Part model, mm, in its own coordinate system. A direction names the side the tool comes from. Round coordinates to 2 decimals unless told otherwise and drop trailing zeros. Order: outer loops, then holes, each group sorted by start corner. A loop starts at its lowest first (then second) coordinate and runs counter-clockwise, first axis right, second up. Notation, with made-up numbers: M -4.5,-32.5 L 23.5,-32.5 A27 cw 23.5,-14.5 Z; hole C 48,22.5 d2. An arc over 180 degrees is marked long. One line per question, with ' | ' between items.
from build123d import *

# Parameters (mm, degrees)
SKETCH1_R           = 17.000673514
SKETCH1_R_2         = 12
BOSS_EXTRUDE1_DEPTH = 15
BOSS_EXTRUDE2_DEPTH = 15
BOSS_EXTRUDE3_DEPTH = 15


with BuildPart() as part:
    # Sketch1 → Boss-Extrude1 (new body)
    with BuildSketch(Plane(origin=(0, 0, 0), x_dir=(1, 0, 0), z_dir=(0, 1, 0))):
        Circle(SKETCH1_R)
        Circle(SKETCH1_R_2, mode=Mode.SUBTRACT)
    extrude(amount=BOSS_EXTRUDE1_DEPTH)

    # Sketch2 → Boss-Extrude2 (add)
    with BuildSketch(Plane(origin=(0, 15, 0), x_dir=(1, 0, 0), z_dir=(0, 1, 0))):
        with BuildLine():
            Line((0, 17.000673514), (25, 17.000673514))
            Line((25, 17.000673514), (25, -17.000673514))
            Line((25, -17.000673514), (0, -17.000673514))
            ThreePointArc((0, -17.000673514), (17.000673514, 0), (0, 17.000673514))
        make_face()
    extrude(amount=-BOSS_EXTRUDE2_DEPTH)

    # Sketch3 → Boss-Extrude3 (add)
    with BuildSketch(Plane(origin=(0, 0, 0), x_dir=(-1, 0, 0), z_dir=(0, -1, 0))):
        with BuildLine():
            ThreePointArc((-29.598035728, 0), (-39.849298386, -24.748737342), (-64.598035728, -35))
            Line((-64.598035728, -35), (-64.598035728, -43.228194221))
            ThreePointArc((-64.598035728, -43.228194221), (-34.031086456, -30.566949272), (-21.369841507, 0))
            ThreePointArc((-21.369841507, 0), (-34.031086456, 30.566949272), (-64.598035728, 43.228194221))
            Line((-64.598035728, 43.228194221), (-64.598035728, 35))
            ThreePointArc((-64.598035728, 35), (-39.849298386, 24.748737342), (-29.598035728, 0))
        make_face()
    extrude(amount=-BOSS_EXTRUDE3_DEPTH)


solid = part.part
1) Saw through at D-D (z = -34). List the corners of the cut face in (x, y), plus the area to 3 significant figures.
The answers:
outline: M 37.9,0 L 56.29,0 L 56.29,15 L 37.9,15 Z | area: 276 mm²
2) Saw through at C-C (x = 21). List the corners of the cut face in (y, z), plus the area to 3 significant figures.
The answers:
outline: M 0,-17 L 15,-17 L 15,17 L 0,17 Z | area: 510 mm²
3) Drop flat-ended pins along their axis: pin 1 (6 mm diameter, centred on x = 52, y = 12, fed in from +Z); pin 2 (8 mm diameter, centred on x = 31.5, y = 9.5, fed in from -Z); pin 3 (1 mm diameter, centred on y = 4.5, z = -32, fed in from -X). Give the stop position or say it passes through.
The answers:
pin 1: stops at z = 42.15 | pin 2: stops at z = -31.97 | pin 3: stops at x = 34.99
4) Two-plate mould, pull along Z, no slides. Class faces 3 (the face through (64.598, 7, -39)), 4 (the face through (-11.99, 7.4, -0.53)), 5 (the face through (13, 8, 17.001)): released by +Z, released by -Z, zero draft, split by the parting line, or undercut.
The answers:
face 3: zero draft | face 4: undercut | face 5: released by +Z
5) Which spindle directions (+Z, -Z, +X, -X, +Y, -Y) get a long thin tool onto all of the face, cutting with end or side? Do faces 1 (the face through (27, 0, 0)), 2 (the face through (12, 8, -17.001)). Say none if no direction does.
The answers:
face 1: +Z, -Z, +X, -X, -Y | face 2: -Z, -X, +Y, -Y
6) Saw through at A-A (x = 55). List the corners of the cut face in (y, z), plus the area to 3 significant figures.
The answers:
outline: M 0,-42.15 L 15,-42.15 L 15,-33.66 L 0,-33.66 Z; M 0,33.66 L 15,33.66 L 15,42.15 L 0,42.15 Z | area: 255 mm²
7) Saw through at B-B (z = -9.5). List the corners of the cut face in (x, y).
The answers:
outline: M -14.1,0 L -7.33,0 L -7.33,15 L -14.1,15 Z; M 7.33,0 L 30.91,0 L 30.91,15 L 7.33,15 Z
8) Probe line 1 (X direction, y = 9.5, z = 0); line 2 (X direction, y = 13, z = -8); line 3 (Z direction, x = 48, y = 0.5). List the from-to ranges inside material, lowest first. Write a range as [from, to].
The answers:
line 1: x = [-17, -12], [12, 29.6] | line 2: x = [-15, -8.94], [8.94, 30.52] | line 3: z = [-39.91, -30.81], [30.81, 39.91]
